Design review of the part built by this model. Coordinates are the model's own, in mm. A direction names the side the tool comes from. Give positions to 0.01 mm unless a question says otherwise; leave off trailing zeros. Loops run counter-clockwise (first coordinate to the right, second up) from the corner with the lowest first, then second, coordinate; pieces in that order, holes last. Notation, with made-up numbers: (48, -9.75) -> (101, -9.75) arc R12 cw to (101, 0.25) -> close; hole circle Ø6 at (77.25, -17). An arc over 180 degrees is marked (long way). Answer in a Markdown table with one row per item. Add a question column.
(1) Consider section A-A on x = -7. Write out the cut boundary in (y, z).
(2) Consider section D-D on y = -12. Write out the cut boundary in (x, z), then the cut area to 3 significant figures.
(3) For faces 5 (the cylindrical face through (0, 2.5, 1.5)), 6 (the flat face through (0, 0, 3)), list the 3-axis set-ups (+Z, -Z, +X, -X, +Y, -Y) from which the entire face can be reached by the end or side of a thin tool; tool diameter is ignored.
(4) For line 1 (Y direction, x = -7, z = 1.85); line 2 (X direction, y = -7.75, z = 0.8); line 3 (X direction, y = -10.75, z = 1.4), list the stretches that pass through material, from the lowest coordinate up.
(5) Draft analysis for pull direction Y (two halves, no side actions). For faces 1 (the cylindrical face through (-8.31, -13, 1.48)), 2 (the flat face through (-0.5, -6, 2)), 3 (the flat face through (0, 15, 1)), 4 (the flat face through (-10, 0, 1)), state which applies: +Y half, -Y half, draft (parallel to the pull), parting line (faces both ways), or undercut.
(6) Consider section C-C on z = 0.9. Write out the cut boundary in (x, y).
(7) Consider section B-B on y = -4.5. Write out the cut boundary in (x, z), then the cut area to 3 significant figures.
from build123d import *

# Parameters (mm, degrees)
CROQUIS1_W              = 20
CROQUIS1_H              = 30
CROQUIS1_R              = 1.65
SALIENTE_EXTRUIR1_DEPTH = 3
CORTAR_EXTRUIR1_REACH   = 5


with BuildPart() as part:
    # Croquis1 → Saliente-Extruir1 (new body)
    with BuildSketch(Plane.XY):
        Rectangle(CROQUIS1_W, CROQUIS1_H)
        with Locations((-7, 12)):
            Circle(CROQUIS1_R, mode=Mode.SUBTRACT)
        with Locations((7, 12)):
            Circle(CROQUIS1_R, mode=Mode.SUBTRACT)
        with Locations((7, -12)):
            Circle(CROQUIS1_R, mode=Mode.SUBTRACT)
        with Locations((-7, -12)):
            Circle(CROQUIS1_R, mode=Mode.SUBTRACT)
    extrude(amount=SALIENTE_EXTRUIR1_DEPTH)

    # Croquis2 → Cortar-Extruir1 (cut, up to next)
    with BuildSketch(Plane.XY.offset(3), mode=Mode.PRIVATE) as cortar_extruir1_sk1:
        with BuildLine():
            Line((-0.5, -9), (-0.5, -3))
            ThreePointArc((-0.5, -3), (0, -2.5), (0.5, -3))
            Line((0.5, -3), (0.5, -9))
            ThreePointArc((0.5, -9), (0, -9.5), (-0.5, -9))
        make_face()
    cortar_extruir1_tool1 = extrude(cortar_extruir1_sk1.sketch, amount=-CORTAR_EXTRUIR1_REACH, mode=Mode.PRIVATE) & part.part
    add(cortar_extruir1_tool1.solids().sort_by_distance((0, -6, 3))[0], mode=Mode.SUBTRACT)
    # Croquis2 → Cortar-Extruir1 (cut, up to next)
    with BuildSketch(Plane.XY.offset(3), mode=Mode.PRIVATE) as cortar_extruir1_sk2:
        with BuildLine():
            Line((-0.5, 3), (-0.5, 9))
            ThreePointArc((-0.5, 9), (0, 9.5), (0.5, 9))
            Line((0.5, 9), (0.5, 3))
            ThreePointArc((0.5, 3), (0, 2.5), (-0.5, 3))
        make_face()
    cortar_extruir1_tool2 = extrude(cortar_extruir1_sk2.sketch, amount=-CORTAR_EXTRUIR1_REACH, mode=Mode.PRIVATE) & part.part
    add(cortar_extruir1_tool2.solids().sort_by_distance((0, 6, 3))[0], mode=Mode.SUBTRACT)


solid = part.part
Values follow:
| question | item | result |
|---|---|---|
| 1 | outline | (-15, 0) -> (-13.65, 0) -> (-13.65, 3) -> (-15, 3) -> close; (-10.35, 0) -> (10.35, 0) -> (10.35, 3) -> (-10.35, 3) -> close; (13.65, 0) -> (15, 0) -> (15, 3) -> (13.65, 3) -> close |
| 2 | outline | (-10, 0) -> (-8.65, 0) -> (-8.65, 3) -> (-10, 3) -> close; (-5.35, 0) -> (5.35, 0) -> (5.35, 3) -> (-5.35, 3) -> close; (8.65, 0) -> (10, 0) -> (10, 3) -> (8.65, 3) -> close |
| 2 | area | 40.2 mm2 |
| 3 | face 5 | +Z, -Z |
| 3 | face 6 | +Z, +X, -X, +Y, -Y |
| 4 | line 1 | -15 to -13.65, -10.35 to 10.35, 13.65 to 15 |
| 4 | line 2 | -10 to -0.5, 0.5 to 10 |
| 4 | line 3 | -10 to -8.08, -5.92 to 5.92, 8.08 to 10 |
| 5 | face 1 | undercut |
| 5 | face 2 | undercut |
| 5 | face 3 | +Y half |
| 5 | face 4 | draft |
| 6 | outline | (-10, -15) -> (10, -15) -> (10, 15) -> (-10, 15) -> close; hole circle Ø3.3 at (-7, -12); hole circle Ø3.3 at (-7, 12); hole (-0.5, -9) arc R0.5 ccw to (0.5, -9) -> (0.5, -3) arc R0.5 ccw to (-0.5, -3) -> close; hole (-0.5, 3) arc R0.5 ccw to (0.5, 3) -> (0.5, 9) arc R0.5 ccw to (-0.5, 9) -> close; hole circle Ø3.3 at (7, -12); hole circle Ø3.3 at (7, 12) |
| 7 | outline | (-10, 0) -> (-0.5, 0) -> (-0.5, 3) -> (-10, 3) -> close; (0.5, 0) -> (10, 0) -> (10, 3) -> (0.5, 3) -> close |
| 7 | area | 57.0 mm2 |
